Work out the finished part from the listing and answer in its coordinate system (mm). Face numbers are marked on the shaded views. A direction names the side the tool comes from. Give positions to 0.01 mm unless a question says otherwise; leave off trailing zeros. Loops run counter-clockwise (first coordinate to the right, second up) from the corner with the lowest first, then second, coordinate; pieces in that order, holes last. Notation, with made-up numbers: M 65,5.25 L 102,5.25 A14 ccw 102,16.25 Z; hole C 10,81 d5. An arc over 180 degrees is marked long. Use a Markdown table: item, result.
```python
from build123d import *

# Parameters (mm, degrees)
SKETCH2_W           = 460
SKETCH2_H           = 460
BOSS_EXTRUDE1_DEPTH = 350
SKETCH3_W           = 460
SKETCH3_H           = 460
BOSS_EXTRUDE2_DEPTH = 150
FILLET1_R           = 70
BOSS_EXTRUDE3_DEPTH = 460
BOSS_EXTRUDE4_REACH = 1254.153


with BuildPart() as part:
    # Sketch2 → Boss-Extrude1 (new body)
    with BuildSketch(Plane(origin=(0, 0, 0), x_dir=(1, 0, 0), z_dir=(0, 1, 0))):
        Rectangle(SKETCH2_W, SKETCH2_H)
    extrude(amount=BOSS_EXTRUDE1_DEPTH)



with BuildPart() as body_2:
    # Sketch3 → Boss-Extrude2 (new body)
    with BuildSketch(Plane(origin=(0, 350, 0), x_dir=(1, 0, 0), z_dir=(0, 1, 0))):
        Rectangle(SKETCH3_W, SKETCH3_H)
    extrude(amount=BOSS_EXTRUDE2_DEPTH)

    # Fillet1
    fillet1_edges = [body_2.edges().sort_by_distance(p)[0] for p in [
        (0, 500, 230),
        (230, 500, 0),
        (0, 500, -230),
        (230, 350, 0),
        (0, 350, 230),
        (-230, 350, 0),
        (0, 350, -230),
        (230, 425, -230),
        (230, 425, 230),
        (-230, 425, 230),
        (-230, 425, -230),
        (-230, 500, 0),
    ]]
    fillet(fillet1_edges, radius=FILLET1_R)


with BuildPart() as part_1:
    add(part.part)

    add(body_2.part)  # Boss-Extrude3 merges body 2
    # Sketch4 → Boss-Extrude3 (add)
    with BuildSketch(Plane.ZY.offset(230)):
        with BuildLine():
            Line((230, 0), (230, 521.319166655))
            ThreePointArc((230, 521.319166655), (282.459718261, 757.839386127), (430, 950))
            ThreePointArc((430, 950), (480, 968.18735527), (530, 950))
            Line((530, 950), (430, 521.319166655))
            Line((430, 521.319166655), (430, 0))
            Line((430, 0), (230, 0))
        make_face()
    extrude(amount=-BOSS_EXTRUDE3_DEPTH)

    # Boss-Extrude4: up to this face of the body (flat: up to its plane)
    boss_extrude4_end = Plane(part_1.part.faces().sort_by_distance((0, 260.659583327, 430))[0])
    # Sketch5 → Boss-Extrude4 (add, up to the picked face)
    with BuildSketch(Plane(origin=(0, 0, -230), x_dir=(-1, 0, 0), z_dir=(0, 0, -1)), mode=Mode.PRIVATE) as boss_extrude4_sk1:
        with BuildLine():
            Line((230, 0), (230, 550))
            ThreePointArc((230, 550), (398.989794856, 659.544511501), (430, 460.5572809))
            ThreePointArc((430, 460.5572809), (393.069360624, 409.991125595), (380, 348.753882025))
            Line((380, 348.753882025), (380, 0))
            Line((380, 0), (230, 0))
        make_face()
    boss_extrude4_tool1 = split(extrude(boss_extrude4_sk1.sketch, amount=-BOSS_EXTRUDE4_REACH, mode=Mode.PRIVATE), bisect_by=boss_extrude4_end, keep=Keep.BOTH, mode=Mode.PRIVATE)
    # Sketch5 → Boss-Extrude4 (add, up to the picked face)
    with BuildSketch(Plane(origin=(0, 0, -230), x_dir=(-1, 0, 0), z_dir=(0, 0, -1)), mode=Mode.PRIVATE) as boss_extrude4_sk2:
        with BuildLine():
            Line((-380, 0), (-230, 0))
            Line((-230, 0), (-230, 550))
            ThreePointArc((-230, 550), (-398.989794856, 659.544511501), (-430, 460.5572809))
            ThreePointArc((-430, 460.5572809), (-393.069360624, 409.991125595), (-380, 348.753882025))
            Line((-380, 348.753882025), (-380, 0))
        make_face()
    boss_extrude4_tool2 = split(extrude(boss_extrude4_sk2.sketch, amount=-BOSS_EXTRUDE4_REACH, mode=Mode.PRIVATE), bisect_by=boss_extrude4_end, keep=Keep.BOTH, mode=Mode.PRIVATE)
    add(boss_extrude4_tool1.solids().sort_by(Axis((-322.302459, 356.474998, -230), (0, 0, 1)))[0])
    add(boss_extrude4_tool2.solids().sort_by(Axis((322.302459, 356.474998, -230), (0, 0, 1)))[0])


solid = part_1.part
```
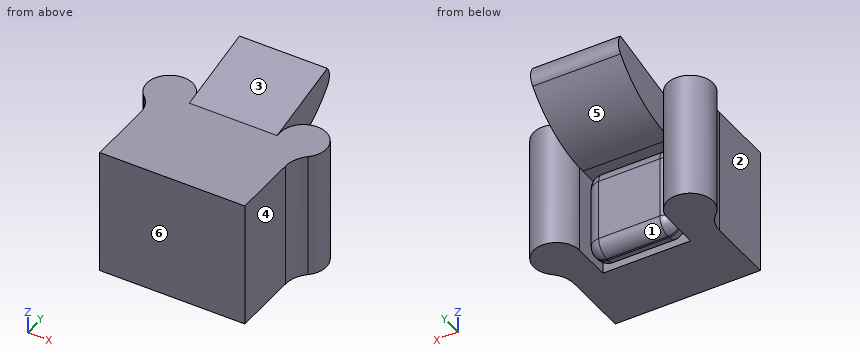
(1) Given P1, Ø4, axis at y = 538, z = 11, coming from the -X side; P2, Ø1.5, axis at y = 367, z = -138, coming from the -X side; P3, Ø5, axis at x = 328, y = 273, coming from the +Z side, each flat-ended and moving along its own axis, determine where each tip first touches the part or whether it passes through.
Entries:
| item | result |
|---|---|
| P1 | stops at x = -469.58 |
| P2 | stops at x = -381.21 |
| P3 | stops at z = 430 |
(2) Which of the six approach directions +Z, -Z, +X, -X, +Y, -Y give full straight-line access (tool end or side, diameter ignored) to the marked faces 1, 2 and 3?
Entries:
| item | result |
|---|---|
| face 1 | -Z, +Y |
| face 2 | +Z, -Z, -X, -Y |
| face 3 | +Z, +X, -X, -Y |
(3) The mould has two halves that part along X. Classify the marked faces 4, 5 and 6: released by +X, released by -X, zero draft, split by the parting line, or undercut.
Entries:
| item | result |
|---|---|
| face 4 | released by +X |
| face 5 | undercut |
| face 6 | zero draft |
(4) A cutting plane is placed at A-A (x = -123.5). Write down the section's boundary in (y, z).
Entries:
| item | result |
|---|---|
| outline | M 0,-230 L 350,-230 L 350,-160 A70 ccw 420,-230 L 430,-230 A70 ccw 500,-160 L 500,160 A70 ccw 430,230 L 521.32,230 A559.42 ccw 950,430 A77.82 ccw 950,530 L 521.32,430 L 0,430 Z; hole M 350,160 A70 cw 420,230 L 350,230 Z |
(5) A cutting plane is placed at D-D (z = 215). Write down the section's boundary in (x, y), and give its area (3 significant figures).
Entries:
| item | result |
|---|---|
| outline | M -430,460.56 A150 cw -380,348.75 L -380,0 L 380,0 L 380,348.75 A150 cw 430,460.56 A120 ccw long 230,550 L 230,350 L -230,350 L -230,550 A120 ccw long Z; M -203.3,420 A43.3 ccw -160,376.7 L 160,376.7 A43.3 ccw 203.3,420 L 203.3,430 A43.3 ccw 160,473.3 L -160,473.3 A43.3 ccw -203.3,430 Z |
| area | 426,000 mm² |
(6) A cutting plane is placed at C-C (y = 387.5). Write down the section's boundary in (x, z), and give its area (3 significant figures).
Entries:
| item | result |
|---|---|
| outline | M -385.09,-230 L -230,-230 L -230,230 L 230,230 L 230,-230 L 385.09,-230 L 385.09,430 L -385.09,430 Z; M -222,-160 A62 ccw -160,-222 L 160,-222 A62 ccw 222,-160 L 222,160 A62 ccw 160,222 L -160,222 A62 ccw -222,160 Z |
| area | 491,000 mm² |
(7) A cutting plane is placed at B-B (z = 107). Write down the section's boundary in (x, y).
Entries:
| item | result |
|---|---|
| outline | M -430,460.56 A150 cw -380,348.75 L -380,0 L 380,0 L 380,348.75 A150 cw 430,460.56 A120 ccw long 230,550 L 230,430 A70 ccw 160,500 L -160,500 A70 ccw -230,430 L -230,550 A120 ccw long Z; hole M -230,350 L -160,350 A70 cw -230,420 Z; hole M 160,350 L 230,350 L 230,420 A70 cw Z |
(8) Consider probe 1 along X at (y, z) = (195, 46); probe 2 along X at (y, z) = (543.5, 238.5); probe 3 along Y at (x, z) = (223.5, -105.5). Determine where each line is inside the solid, lowest interval first. Write a range as [from, to].
Entries:
| item | result |
|---|---|
| probe 1 | x = [-380, 380] |
| probe 2 | x = [-469.82, 469.82] |
| probe 3 | y = [0, 350], [390.54, 459.46] |
